```python
from build123d import *

# Parameters (mm, degrees)
SKETCH4_R           = 3.81
SKETCH4_R_2         = 3.048
BOSS_EXTRUDE1_DEPTH = 2.54
SKETCH4_3_R         = 3.81
SKETCH4_3_R_2       = 3.048


with BuildPart() as part:
    # Sketch4 → Boss-Extrude1 (new body)
    with BuildSketch(Plane(origin=(0, 110.370938621, 0), x_dir=(-1, 0, 0), z_dir=(0, 1, 0))):
        Circle(SKETCH4_R)
        Circle(SKETCH4_R_2, mode=Mode.SUBTRACT)
    extrude(amount=-BOSS_EXTRUDE1_DEPTH)

    # Sweep2: sweep along a path in Sketch3
    with BuildLine(Plane.XY) as sweep2_path:
        Line((0, 110.370938621), (0, 81.839949684))
        ThreePointArc((0, 81.839949684), (19.796310895, 33.11982338), (67.964229263, 12.015409809))
        Line((67.964229263, 12.015409809), (93.926499612, 11.314239564))
    # Sketch4<3> → Sweep2 (sweep)
    with BuildSketch(Plane(origin=(0, 110.370938621, 0), x_dir=(-1, 0, 0), z_dir=(0, 1, 0))):
        Circle(SKETCH4_3_R)
        Circle(SKETCH4_3_R_2, mode=Mode.SUBTRACT)
    sweep(path=sweep2_path.line)


solid = part.part
```
Geometry check sheet. Reference: the model listing, model coordinates, mm. A direction names the side the tool comes from. Coordinates: 2 decimals unless noted, no trailing zeros. Order: outer loops, then holes, each group sorted by start corner. A loop starts at its lowest first (then second) coordinate and runs counter-clockwise, first axis right, second up. Notation, with made-up numbers: (66, 10) - (119, 10) arc R22 ccw to (119, 32) - close; hole circle Ø9 at (-6.75, -10.75). An arc over 180 degrees is marked (long way). Answer as a JSON object with one key per item and string values. Group by question number.
Item 1: Scan lines: probe 1 along X at (y, z) = (96.25, 0); probe 2 along X at (y, z) = (37, 2). Record each from-to range of solid material in increasing order.
Item 2: Draft check along Z on faces 3 (the face through (2, 110.371, 3)), 4 (the face through (81.049, 8.754, -0.916)), 5 (the face through (0.83, 96.31, -3.72)). Enter one of: +Z half, -Z half, draft (parallel to the pull), parting line (faces both ways), or undercut.
Item 3: Sectioned sample at A-A, the plane z = 1.75. Record the cut outline in (x, y).
Item 4: Sectioned sample at B-B, the plane y = 98. Record the cut outline in (x, z), and give its area (3 significant figures).
Item 5: Depth check by flat-ended pin: pin 1 Ø4 at (x, z) = (70, -1) entering from -Y; pin 2 Ø4 at (x, z) = (32, -2) entering from -Y; pin 3 Ø2 at (y, z) = (93, 2) entering from -X. Enter the tip coordinate at first touch or a pass-through.
Item 6: Tool access check on faces 1 (the face through (81.03, 8.14, 1.46)), 2 (the face through (0.4, 96.31, 3.02)). Record the directions out of +Z, -Z, +X, -X, +Y, -Y that give a thin tool (end or side, any length) a straight path to the whole face; none if there is none.
Resolved:
{
 "1": {"probe 1": "-3.81 to -3.05, 3.05 to 3.81", "probe 2": "12.13 to 13.33, 19.33 to 20.6"},
 "2": {"face 3": "draft", "face 4": "undercut", "face 5": "parting line"},
 "3": {"outline": "(-3.38, 81.84) arc R73.23 ccw to (67.87, 8.63) - (93.84, 7.93) - (93.86, 8.82) - (67.9, 9.52) arc R72.35 cw to (-2.5, 81.84) - (-2.5, 110.37) - (-3.38, 110.37) - close; (2.5, 81.84) arc R67.35 ccw to (68.03, 14.51) - (93.99, 13.81) - (94.02, 14.7) - (68.06, 15.4) arc R66.47 cw to (3.38, 81.84) - (3.38, 110.37) - (2.5, 110.37) - close"},
 "4": {"outline": "circle Ø7.62 at (0, 0); hole circle Ø6.1 at (0, 0)", "area": "16.4 mm^2"},
 "5": {"pin 1": "y = 8.1", "pin 2": "y = 17.8", "pin 3": "x = -3.68"},
 "6": {"face 1": "none", "face 2": "+Y"}
}
